The listing builds one solid part. Answer for the finished solid, in the listing's coordinates (mm). Face numbers are marked on the shaded views. Round coordinates to 2 decimals unless told otherwise and drop trailing zeros. Loops run counter-clockwise (first coordinate to the right, second up) from the corner with the lowest first, then second, coordinate; pieces in that order, holes last. Notation, with made-up numbers: (58.5, -10) -> (64.5, -10) arc R19 cw to (64.5, 13) -> close; hole circle Ø3 at (78, 74.5). An arc over 180 degrees is marked (long way). Use a Markdown table: item, result. Add a question column.
Q1. Section A-A on z = 15.98 is taken. Give the vertices of the cut face in (x, y), then the cut area to 3 significant figures.
Q2. Given pin 1 Ø5 at (x, z) = (282.5, 10) entering from +Y; pin 2 Ø5 at (x, z) = (283, 10) entering from -Y; pin 3 Ø3 at (y, z) = (-41.87, 15.98) entering from -X, each flat-ended and moving along its own axis, determine where each tip first touches the part or whether it passes through.
Q3. Consider line 1 (X direction, y = -94.5, z = -0.5); line 2 (Y direction, x = 284.6, z = 15.98); line 3 (Y direction, x = 279, z = 6). Determine where each line is inside the solid, lowest interval first.
Q4. Section B-B on y = -109 is taken. Give the vertices of the cut face in (x, z).
Q5. Section C-C on x = 246.5 is taken. Give the vertices of the cut face in (y, z), then the cut area to 3 significant figures.
Q6. For a pull along X with two mould halves and no side action, classify the marked faces 1 and 2 as released by +X, released by -X, zero draft, split by the parting line, or undercut.
from build123d import *

# Parameters (mm, degrees)
BOSS_EXTRUDE1_DEPTH      = 2.54
SKETCH2_W                = 74.651204731
SKETCH2_H                = 103.727
BOSS_EXTRUDE2_DEPTH      = 2
CAMERA_RIBBON_HOLE_DEPTH = 4.54
SKETCH4_W                = 29
SKETCH4_H                = 31.8
RFD900_HOLE_DEPTH        = 3.5
SKETCH5_R                = 2.7
SKETCH5_R_2              = 1.45
RFD900_MOUNT_DEPTH       = 2.784999988
WIRE_START               = -2
SKETCH6_W                = 8.202097681
SKETCH6_H                = 71.209120783
WIRE_HOLE_DEPTH          = 4.54
SKETCH7_W                = 6.492515401
SKETCH7_H                = 6.35
BOSS_EXTRUDE4_DEPTH      = 17.36
CUT_EXTRUDE4_REACH       = 300.389
SKETCH13_R               = 1.375000001
CUT_EXTRUDE7_DEPTH       = 2.535264343
CUT_EXTRUDE6_START       = -4.54
SKETCH12_R               = 1.45
CUT_EXTRUDE6_DEPTH       = 4.54
SKETCH15_R               = 1.9
CUT_EXTRUDE8_DEPTH       = 4.54
SKETCH16_R               = 1.375
CUT_EXTRUDE9_DEPTH       = 4.54


with BuildPart() as part:
    # Sketch1 → Boss-Extrude1 (new body)
    with BuildSketch(Plane.XY):
        with BuildLine():
            Line((209.003679248, -17.464278872), (283.585283979, -17.464278872))
            ThreePointArc((283.585283979, -17.464278872), (284.698835738, -17.925527113), (285.160083979, -19.039078872))
            Line((285.160083979, -19.039078872), (285.160083979, -122.696478872))
            ThreePointArc((285.160083979, -122.696478872), (284.698835738, -123.810030631), (283.585283979, -124.271278872))
            Line((283.585283979, -124.271278872), (209.003679248, -124.271278872))
            ThreePointArc((209.003679248, -124.271278872), (207.890127489, -123.810030631), (207.428879248, -122.696478872))
            Line((207.428879248, -122.696478872), (207.428879248, -19.039078872))
            ThreePointArc((207.428879248, -19.039078872), (207.890127489, -17.925527113), (209.003679248, -17.464278872))
        make_face()
    extrude(amount=BOSS_EXTRUDE1_DEPTH)

    # Sketch2 → Boss-Extrude2 (add)
    with BuildSketch(Plane(origin=(0, 0, 0), x_dir=(-1, 0, 0), z_dir=(0, 0, -1))):
        with Locations((-246.294481614, -70.867778872)):
            Rectangle(SKETCH2_W, SKETCH2_H)
    extrude(amount=BOSS_EXTRUDE2_DEPTH)

    # Sketch3 → Camera Ribbon Hole (cut)
    with BuildSketch(Plane.XY.offset(2.54)):
        with BuildLine():
            Line((214.972517673, -105.55645249), (231.085240907, -105.55645249))
            ThreePointArc((231.085240907, -105.55645249), (231.52887929, -106.906363326), (230.265368958, -107.55645249))
            Line((230.265368958, -107.55645249), (215.792389622, -107.55645249))
            ThreePointArc((215.792389622, -107.55645249), (214.52887929, -106.906363326), (214.972517673, -105.55645249))
        make_face()
    extrude(amount=-CAMERA_RIBBON_HOLE_DEPTH, mode=Mode.SUBTRACT)

    # Sketch4 → RFD900 Hole (cut)
    with BuildSketch(Plane.XY.offset(2.54)):
        with Locations((233.09754244, -88.65645249)):
            Rectangle(SKETCH4_W, SKETCH4_H)
    extrude(amount=-RFD900_HOLE_DEPTH, mode=Mode.SUBTRACT)

    # Sketch5 → RFD900 Mount (add)
    # profile 1 of 3: a face of its own
    with BuildSketch(Plane.XY.offset(2.54)):
        with Locations(Location((215.071008708, -88.65645249, 0), (0, 0, 180))):
            Circle(SKETCH5_R)
        with Locations((215.071008708, -88.65645249)):
            Circle(SKETCH5_R_2, mode=Mode.SUBTRACT)
    # profile 2 of 3: a face of its own
    with BuildSketch(Plane.XY.offset(2.54)):
        with Locations(Location((252.671008708, -101.20645249, 0), (0, 0, 180))):
            Circle(SKETCH5_R)
        with Locations((252.671008708, -101.20645249)):
            Circle(SKETCH5_R_2, mode=Mode.SUBTRACT)
    # profile 3 of 3: a face of its own
    with BuildSketch(Plane.XY.offset(2.54)):
        with Locations(Location((252.671008708, -76.10645249, 0), (0, 0, 180))):
            Circle(SKETCH5_R)
        with Locations((252.671008708, -76.10645249)):
            Circle(SKETCH5_R_2, mode=Mode.SUBTRACT)
    extrude(amount=RFD900_MOUNT_DEPTH)

    # Sketch6 → Wire Hole (cut)
    with BuildSketch(Plane.XY.offset(WIRE_START)):
        with Locations((274.024654874, -70.867778873)):
            Rectangle(SKETCH6_W, SKETCH6_H)
    extrude(amount=WIRE_HOLE_DEPTH, mode=Mode.SUBTRACT)

    # Sketch7 → Boss-Extrude4 (add)
    with BuildSketch(Plane.XY.offset(2.54)):
        with Locations((281.913826279, -41.867778872)):
            Rectangle(SKETCH7_W, SKETCH7_H)
        with Locations((281.913826279, -99.867778872)):
            Rectangle(SKETCH7_W, SKETCH7_H)
    extrude(amount=BOSS_EXTRUDE4_DEPTH)

    # Cut-Extrude4: up to this face of the body (flat: up to its plane)
    cut_extrude4_end = Plane(part.part.faces().sort_by_distance((281.913826279, -38.692778872, 11.22))[0])
    # Sketch8 → Cut-Extrude4 (cut, up to the picked face)
    with BuildSketch(Plane.XZ.offset(103.042778872), mode=Mode.PRIVATE) as cut_extrude4_sk1:
        Polygon((282.624819635, 11.684999999), (278.667568578, 7.727748942), (278.667568578, 19.9), (282.624819635, 19.9), (282.624819635, 16.98), (282.624819635, 14.604999999), align=None)
    cut_extrude4_tool1 = split(extrude(cut_extrude4_sk1.sketch, amount=-CUT_EXTRUDE4_REACH, mode=Mode.PRIVATE), bisect_by=cut_extrude4_end, keep=Keep.BOTH, mode=Mode.PRIVATE)
    add(cut_extrude4_tool1.solids().sort_by(Axis((280.518174, -103.042779, 14.739177), (0, 1, 0)))[0], mode=Mode.SUBTRACT)

    # Sketch13 → Cut-Extrude7 (cut)
    with BuildSketch(Plane(origin=(285.160083979, 0, 0), x_dir=(0, 0, -1), z_dir=(1, 0, 0))):
        with Locations((-15.98, -99.867778872)):
            Circle(SKETCH13_R)
        with Locations((-15.98, -41.867778872)):
            Circle(SKETCH13_R)
    extrude(amount=-CUT_EXTRUDE7_DEPTH, mode=Mode.SUBTRACT)

    # Sketch12 → Cut-Extrude6 (cut)
    with BuildSketch(Plane.XY.offset(2.54).offset(CUT_EXTRUDE6_START)):
        with Locations(Location((252.671008708, -76.10645249, 0), (0, 0, 180))):
            Circle(SKETCH12_R)
        with Locations(Location((252.671008708, -101.20645249, 0), (0, 0, 180))):
            Circle(SKETCH12_R)
        with Locations(Location((215.071008708, -88.65645249, 0), (0, 0, 180))):
            Circle(SKETCH12_R)
    extrude(amount=CUT_EXTRUDE6_DEPTH, mode=Mode.SUBTRACT)

    # Sketch15 → Cut-Extrude8 (cut)
    with BuildSketch(Plane.XY.offset(2.54)):
        with Locations((213.103879248, -23.139278872)):
            Circle(SKETCH15_R)
        with Locations((259.103879248, -23.139278872)):
            Circle(SKETCH15_R)
        with Locations((213.103879248, -69.139278872)):
            Circle(SKETCH15_R)
        with Locations((259.103879248, -69.139278872)):
            Circle(SKETCH15_R)
    extrude(amount=-CUT_EXTRUDE8_DEPTH, mode=Mode.SUBTRACT)

    # Sketch16 → Cut-Extrude9 (cut)
    with BuildSketch(Plane.XY.offset(2.54)):
        with Locations((228.028879248, -112.696478872)):
            Circle(SKETCH16_R)
        with Locations((223.028879248, -117.696478872)):
            Circle(SKETCH16_R)
        with Locations((218.028879248, -112.696478872)):
            Circle(SKETCH16_R)
    extrude(amount=-CUT_EXTRUDE9_DEPTH, mode=Mode.SUBTRACT)


solid = part.part
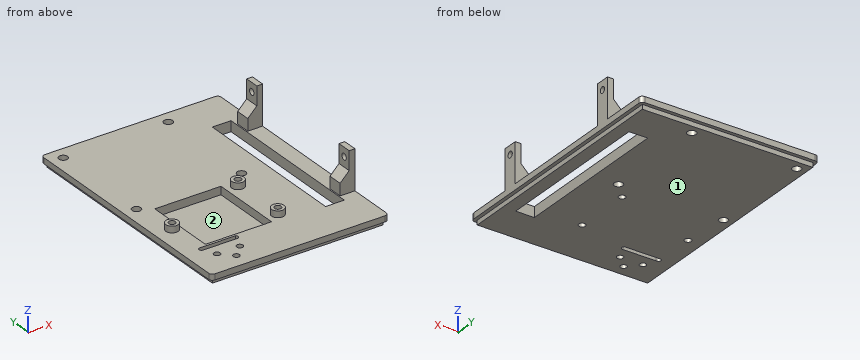
Checked values:
| question | item | result |
|---|---|---|
| 1 | outline | (282.62, -103.04) -> (285.16, -103.04) -> (285.16, -101.24) -> (282.62, -101.24) -> close; (282.62, -98.49) -> (285.16, -98.49) -> (285.16, -96.69) -> (282.62, -96.69) -> close; (282.62, -45.04) -> (285.16, -45.04) -> (285.16, -43.24) -> (282.62, -43.24) -> close; (282.62, -40.49) -> (285.16, -40.49) -> (285.16, -38.69) -> (282.62, -38.69) -> close |
| 1 | area | 18.3 mm2 |
| 2 | pin 1 | stops at y = -38.69 |
| 2 | pin 2 | stops at y = -103.04 |
| 2 | pin 3 | stops at x = 282.62 |
| 3 | line 1 | x = 208.97 to 218.6, 247.6 to 269.92, 278.13 to 283.62 |
| 3 | line 2 | y = -103.04 to -101.24, -98.49 to -96.69, -45.04 to -43.24, -40.49 to -38.69 |
| 3 | line 3 | y = -103.04 to -96.69, -45.04 to -38.69 |
| 4 | outline | (207.43, 0) -> (208.97, 0) -> (208.97, -2) -> (283.62, -2) -> (283.62, 0) -> (285.16, 0) -> (285.16, 2.54) -> (207.43, 2.54) -> close |
| 5 | outline | (-124.27, 0) -> (-122.73, 0) -> (-122.73, -2) -> (-19, -2) -> (-19, 0) -> (-17.46, 0) -> (-17.46, 2.54) -> (-72.76, 2.54) -> (-72.76, -0.96) -> (-104.56, -0.96) -> (-104.56, 2.54) -> (-124.27, 2.54) -> close |
| 5 | area | 367 mm2 |
| 6 | face 1 | zero draft |
| 6 | face 2 | undercut |
